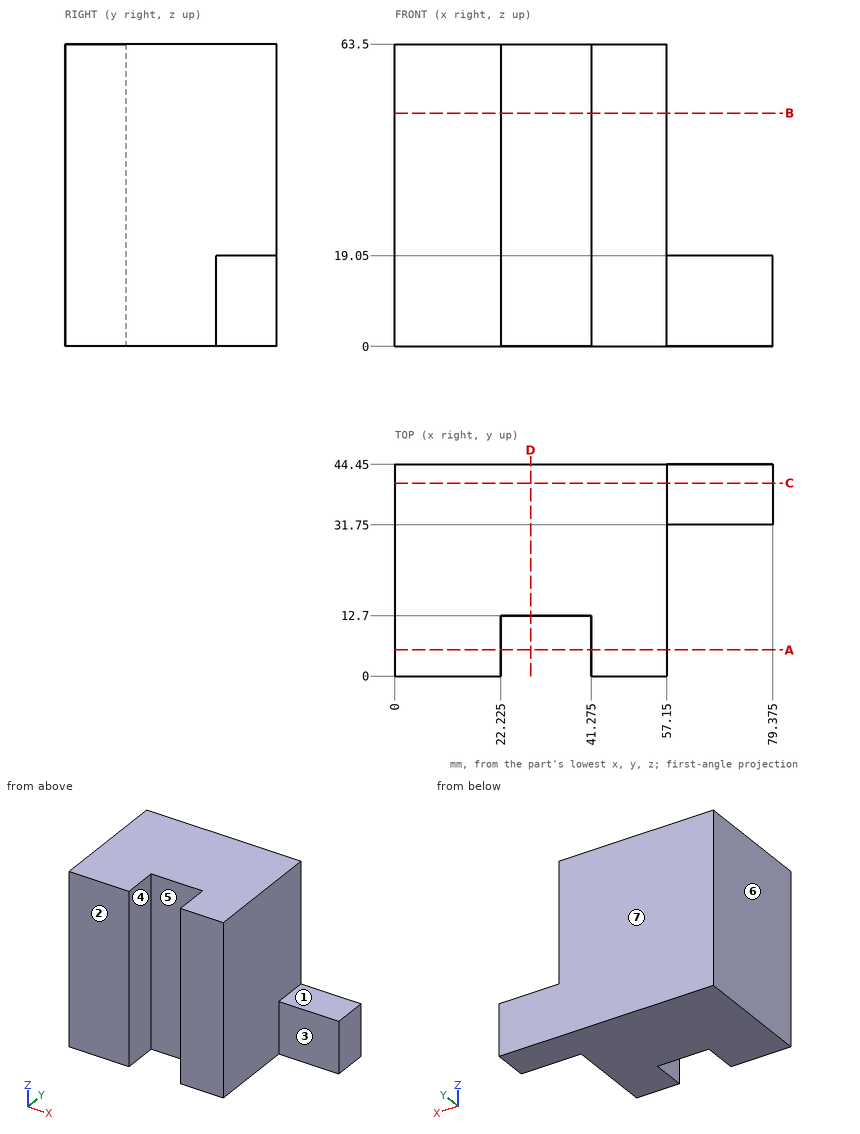
Part print with two shaded views. Sizes in mm from the minimum x, y, z corner. A direction names the side the tool comes from. Coordinates: 2 decimals unless noted, no trailing zeros. Write each loop counter-clockwise with the first axis right and the second up, starting at its lowest first coordinate (ties: lowest second). Pieces come first, ordered by that corner, then holes. Notation, with made-up numbers: (57.25, -16.5) - (89.25, -16.5) arc R19 cw to (89.25, -4.5) - close; hole circle Ø1 at (45.25, 54). An arc over 180 degrees is marked (long way). Put each result on its own line as item: value.
1. Band-saw the part on D-D (x = 28.5). Write the cut outline in (y, z), then the cut area to 3 significant figures.
Final values:
outline: (12.7, 0) - (44.45, 0) - (44.45, 63.5) - (12.7, 63.5) - close
area: 2,020 mm²
2. Two-plate mould, pull along X, no slides. Class the marked faces 4, 5, 6 and 7: +X half, -X half, draft (parallel to the pull), parting line (faces both ways), or undercut.
Final values:
face 4: undercut
face 5: undercut
face 6: -X half
face 7: draft
3. 3-axis set-ups, long thin cutter, end or side, ignore diameter. For the marked faces 1, 2 and 3: which of +Z, -Z, +X, -X, +Y, -Y reach the whole face in a straight line?
Final values:
face 1: +Z, +X, +Y, -Y
face 2: +Z, -Z, +X, -X, -Y
face 3: +Z, -Z, +X, -Y
4. Band-saw the part on C-C (y = 40.5). Write the cut outline in (x, z) (3 decimals).
Final values:
outline: (0, 0) - (79.375, 0) - (79.375, 19.05) - (57.15, 19.05) - (57.15, 63.5) - (0, 63.5) - close
5. Flat gauge pins, fed straight in: pin 1 Ø21 at (x, z) = (68, 12) entering from -Y; pin 2 Ø13.5 at (y, z) = (12.5, 42) entering from +X; pin 3 Ø14 at (x, y) = (73.5, 38) entering from +Z; pin 4 Ø10 at (y, z) = (7, 23) entering from -X. Where does each tip first touch, or does it go through?
Final values:
pin 1: stops at y = 31.75
pin 2: stops at x = 57.15
pin 3: stops at z = 19.05
pin 4: stops at x = 0
6. Probe line 1 along X through (y, z) = (12.5, 49) (3 decimals); line 2 along Y through (x, z) = (34, 5); line 3 along X through (y, z) = (24.5, 20). List the from-to ranges inside material, lowest first. Write a range as [from, to].
Final values:
line 1: x = [0, 22.225], [41.275, 57.15]
line 2: y = [12.7, 44.45]
line 3: x = [0, 57.15]
7. Band-saw the part on A-A (y = 5.5). Write the cut outline in (x, z) (3 decimals), then the cut area to 3 significant figures.
Final values:
outline: (0, 0) - (22.225, 0) - (22.225, 63.5) - (0, 63.5) - close; (41.275, 0) - (57.15, 0) - (57.15, 63.5) - (41.275, 63.5) - close
area: 2,420 mm²
8. Band-saw the part on B-B (z = 49). Write the cut outline in (x, y) (3 decimals).
Final values:
outline: (0, 0) - (22.225, 0) - (22.225, 12.7) - (41.275, 12.7) - (41.275, 0) - (57.15, 0) - (57.15, 44.45) - (0, 44.45) - close
